from build123d import *

# Parameters (mm, degrees)
BOSS_EXTRUDE1_DEPTH = 1.5875
SKETCH2_W           = 10.414
SKETCH2_H           = 0.635
SKETCH2_W_2         = 19.558
SKETCH2_W_3         = 7.3914
SKETCH2_H_2         = 0.889
CUT_EXTRUDE1_DEPTH  = 56.607220803
SKETCH3_W           = 31.75
SKETCH3_H           = 0.635
CUT_EXTRUDE3_DEPTH  = 56.607220803


with BuildPart() as part:
    # Sketch1 → Boss-Extrude1 (new, symmetric)
    with BuildSketch(Plane(origin=(0, 0, 0), x_dir=(1, 0, 0), z_dir=(0, 1, 0))):
        Polygon((-49.022, -7.3025), (-49.022, 7.3025), (-51.943, 7.3025), (-51.943, 13.9065), (-41.529, 13.9065), (-41.529, 16.7259), (-9.779, 16.7259), (-9.779, 13.9065), (9.779, 13.9065), (9.779, 16.7259), (41.529, 16.7259), (41.529, 14.1605), (48.9204, 14.1605), (48.9204, 7.3025), (51.8414, 7.3025), (51.8414, -7.3025), (48.9204, -7.3025), (48.9204, -14.1605), (41.529, -14.1605), (41.527983985, -19.596099905), (9.779, -19.3421), (9.779, -13.9065), (-9.779, -13.9065), (-9.779, -19.3421), (-41.529, -19.3421), (-41.529, -13.9065), (-51.943, -13.9065), (-51.943, -7.3025), align=None)
    extrude(amount=BOSS_EXTRUDE1_DEPTH, both=True)

    # Sketch2 → Cut-Extrude1 (cut, through all)
    with BuildSketch(Plane(origin=(0, 1.5875, 0), x_dir=(1, 0, 0), z_dir=(0, 1, 0))):
        with Locations((-46.736, 13.589)):
            Rectangle(SKETCH2_W, SKETCH2_H)
        with Locations((0, 13.589)):
            Rectangle(SKETCH2_W_2, SKETCH2_H)
        with Locations((45.2247, 13.716)):
            Rectangle(SKETCH2_W_3, SKETCH2_H_2)
    extrude(amount=-CUT_EXTRUDE1_DEPTH, mode=Mode.SUBTRACT)

    # Sketch3 → Cut-Extrude3 (cut, through all)
    with BuildSketch(Plane(origin=(0, 1.5875, 0), x_dir=(1, 0, 0), z_dir=(0, 1, 0))):
        with Locations((-25.654, 16.4084)):
            Rectangle(SKETCH3_W, SKETCH3_H)
        Polygon((9.779, -19.3421), (41.528031462, -19.3421), (41.527983985, -19.596099905), (9.779096987, -19.596099905), align=None)
        with Locations((25.654, 16.4084)):
            Rectangle(SKETCH3_W, SKETCH3_H)
    extrude(amount=-CUT_EXTRUDE3_DEPTH, mode=Mode.SUBTRACT)


solid = part.part
Here's how the part is built. I have some questions about the finished solid (model axes, mm). A direction names the side the tool comes from. Give positions to 0.01 mm unless a question says otherwise; leave off trailing zeros. Loops run counter-clockwise (first coordinate to the right, second up) from the corner with the lowest first, then second, coordinate; pieces in that order, holes last. Notation, with made-up numbers: (63.5, 71) -> (78.5, 71) arc R20 ccw to (78.5, 87) -> close; hole circle Ø8 at (70.25, 57.25). An arc over 180 degrees is marked (long way). Answer as a JSON object with one key per item and string values. Group by question number.
Item 1: Thinking about a two-plate mould opening in Z: for faces 6 (the flat face through (-49.022, 0, 0)), 7 (the flat face through (25, 0, 19.342)), 8 (the flat face through (9.779, 0, -15)), 9 (the flat face through (-26, 0, -16.091)), which applies, pulls with the +Z half, pulls with the -Z half, needs draft (parallel to the pull), parting line crosses it, or undercut?
Item 2: I need wall thicknesses on L1, parallel to X at y = 0.7, z = 17.5; L2, parallel to X at y = -1, z = -13; L3, parallel to Z at x = -2, y = -0.35. Which ranges of each line are inside material? Lowest first, please.
Item 3: Imagine slicing it at A-A on y = 0.4. Write out the boundary of the cut face in (x, z), then the cut area to 3 significant figures.
Item 4: Will these pins go through, and if not, where does the flat tip stop? pin 1 (1.4 mm diameter, centred on y = -0.5, z = -14.5, fed in from -X); pin 2 (1 mm diameter, centred on x = -45, y = -0.5, fed in from -Z); pin 3 (1 mm diameter, centred on y = 0.5, z = 10.5, fed in from +X).
Item 5: Imagine slicing it at C-C on z = -4. Write out the boundary of the cut face in (x, y).
Item 6: Imagine slicing it at B-B on x = 7.5. Write out the boundary of the cut face in (y, z), then the cut area to 3 significant figures.
Item 7: On a 3-axis mill with a long thin cutter (end or side, diameter ignored), from which of +Z, -Z, +X, -X, +Y, -Y can I reach the whole of each face in a straight line? I mean faces 1 (the flat face through (-51, 0, 7.302)), 2 (the flat face through (-41.529, 0, 17)), 3 (the flat face through (48.92, 0, 11)), 4 (the flat face through (48.92, 0, -10)), 5 (the flat face through (0, 0, 13.906)). Say none if no direction works.
Answer list:
{
 "1": {"face 6": "undercut", "face 7": "pulls with the +Z half", "face 8": "needs draft", "face 9": "pulls with the -Z half"},
 "2": {"L1": "x = -41.53 to -9.78, 9.78 to 41.53", "L2": "x = -51.94 to 48.92", "L3": "z = -13.27 to 13.91"},
 "3": {"outline": "(-51.94, -13.27) -> (-41.53, -13.27) -> (-41.53, -16.09) -> (-9.78, -16.09) -> (-9.78, -13.27) -> (9.78, -13.27) -> (9.78, -16.09) -> (41.53, -16.09) -> (41.53, -13.27) -> (48.92, -13.27) -> (48.92, -7.3) -> (51.84, -7.3) -> (51.84, 7.3) -> (48.92, 7.3) -> (48.92, 14.16) -> (41.53, 14.16) -> (41.53, 19.34) -> (9.78, 19.34) -> (9.78, 13.91) -> (-9.78, 13.91) -> (-9.78, 19.34) -> (-41.53, 19.34) -> (-41.53, 13.91) -> (-51.94, 13.91) -> (-51.94, 7.3) -> (-49.02, 7.3) -> (-49.02, -7.3) -> (-51.94, -7.3) -> close", "area": "3,270 mm2"},
 "4": {"pin 1": "stops at x = -41.53", "pin 2": "stops at z = -13.27", "pin 3": "stops at x = 48.92"},
 "5": {"outline": "(-49.02, -1.59) -> (51.84, -1.59) -> (51.84, 1.59) -> (-49.02, 1.59) -> close"},
 "6": {"outline": "(-1.59, -13.27) -> (1.59, -13.27) -> (1.59, 13.91) -> (-1.59, 13.91) -> close", "area": "86.3 mm2"},
 "7": {"face 1": "-X, +Y, -Y", "face 2": "+Z, -X, +Y, -Y", "face 3": "+Z, +X, +Y, -Y", "face 4": "-Z, +X, +Y, -Y", "face 5": "+Z, +Y, -Y"}
}
